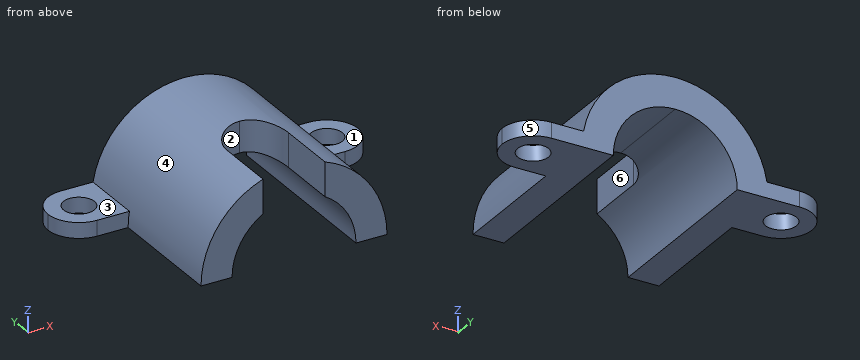
```python
from build123d import *

# Parameters (mm, degrees)
F1_W      = 60
F1_H      = 60
F2_DEPTH  = 30
F4_DEPTH  = 60.001
F5_W      = 20
F5_H      = 20
F6_DEPTH  = 5
F7_W      = 20
F7_H      = 20
F8_DEPTH  = 5
F10_DEPTH = 20
F12_DEPTH = 40
F13_R     = 9.99999
F14_R     = 9.99999
F15_R     = 5
F16_DEPTH = 5.001
F17_R     = 5
F18_DEPTH = 5.001
F20_DEPTH = 30
F21_R     = 10
F22_R     = 9.99999


# Not quite as in the source:
# - a fillet or chamfer is up to 0.001 mm smaller than in the source, because OpenCascade refuses the exact size


with BuildPart() as f2:
    # F1 (on Top) → F2 (new body)
    with BuildSketch(Plane.XY):
        Rectangle(F1_W, F1_H)
    extrude(amount=F2_DEPTH)

    # F3 (on face) → F4 (cut, through all)
    with BuildSketch(Plane.XZ.offset(30)):
        with BuildLine():
            ThreePointArc((20, 0), (14.1421356237, 14.1421356237), (0, 20))
            Line((0, 20), (0, 0))
            Line((0, 0), (20, 0))
        make_face()
        with BuildLine():
            Line((0, 0), (0, 20))
            ThreePointArc((0, 20), (-14.1421356237, 14.1421356237), (-20, 0))
            Line((-20, 0), (0, 0))
        make_face()
    extrude(amount=-F4_DEPTH, mode=Mode.SUBTRACT)

    # F5 (on Top) → F6 (join)
    with BuildSketch(Plane.XY):
        with Locations((40, 20)):
            Rectangle(F5_W, F5_H)
    extrude(amount=F6_DEPTH)

    # F7 (on Top) → F8 (join)
    with BuildSketch(Plane.XY):
        with Locations((-40, 20)):
            Rectangle(F7_W, F7_H)
    extrude(amount=F8_DEPTH)

    # F9 (on face) → F10 (cut)
    with BuildSketch(Plane(origin=(0, 30, 0), x_dir=(-1, 0, 0), z_dir=(0, 1, 0))):
        with BuildLine():
            ThreePointArc((-29.5803989155, 5), (-19.3649167147, 22.9128784886), (4.28e-08, 30))
            Line((4.28e-08, 30), (-30, 30))
            Line((-30, 30), (-30, 5))
            Line((-30, 5), (-29.5803989155, 5))
        make_face()
        with BuildLine():
            ThreePointArc((4.28e-08, 30), (19.3649167474, 22.912878461), (29.5803989155, 5))
            Line((29.5803989155, 5), (30, 5))
            Line((30, 5), (30, 30))
            Line((30, 30), (4.28e-08, 30))
        make_face()
    extrude(amount=-F10_DEPTH, mode=Mode.SUBTRACT)

    # F11 (on face) → F12 (cut)
    with BuildSketch(Plane.XZ.offset(30)):
        with BuildLine():
            Line((-30, 30), (-30, 0))
            ThreePointArc((-30, 0), (-21.2132034683, 21.2132034029), (-9.24e-08, 30))
            Line((-9.24e-08, 30), (-30, 30))
        make_face()
        with BuildLine():
            ThreePointArc((-9.24e-08, 30), (21.2132034029, 21.2132034683), (30, 0))
            Line((30, 0), (30, 30))
            Line((30, 30), (-9.24e-08, 30))
        make_face()
    extrude(amount=-F12_DEPTH, mode=Mode.SUBTRACT)

    # F13 (radius 10 in the source; OpenCascade refuses exactly that, so slightly less here)
    f13_edges = [f2.edges().sort_by_distance(p)[0] for p in [
        (50, 30, 2.5),
        (50, 10, 2.5),
    ]]
    fillet(f13_edges, radius=F13_R)

    # F14 (radius 10 in the source; OpenCascade refuses exactly that, so slightly less here)
    f14_edges = [f2.edges().sort_by_distance(p)[0] for p in [
        (-50, 30, 2.5),
        (-50, 10, 2.5),
    ]]
    fillet(f14_edges, radius=F14_R)

    # F15 (on face) → F16 (cut, through all)
    with BuildSketch(Plane.XY.offset(5)):
        with Locations((-40, 20)):
            Circle(F15_R)
    extrude(amount=-F16_DEPTH, mode=Mode.SUBTRACT)

    # F17 (on face) → F18 (cut, through all)
    with BuildSketch(Plane.XY.offset(5)):
        with Locations((40, 20)):
            Circle(F17_R)
    extrude(amount=-F18_DEPTH, mode=Mode.SUBTRACT)

    # F19 (on face) → F20 (cut)
    with BuildSketch(Plane.XZ.offset(30)):
        with BuildLine():
            Line((10, 17.3205080757), (10, 28.2842712437))
            ThreePointArc((10.0000000012, 28.284271247), (1.3e-09, 30), (-9.9999999988, 28.2842712479))
            Line((-10, 28.2842712513), (-10, 17.3205080757))
            ThreePointArc((-10, 17.3205080757), (0, 20), (10, 17.3205080757))
        make_face()
    extrude(amount=-F20_DEPTH, mode=Mode.SUBTRACT)

    # F21
    f21_edges = [f2.edges().sort_by_distance(p)[0] for p in [
        (-10, 0, 22.80239),
    ]]
    fillet(f21_edges, radius=F21_R)

    # F22 (radius 10 in the source; OpenCascade refuses exactly that, so slightly less here)
    f22_edges = [f2.edges().sort_by_distance(p)[0] for p in [
        (10, 0, 22.80239),
    ]]
    fillet(f22_edges, radius=F22_R)


solid = f2.part
```
Part model, mm, in its own coordinate system. Face numbers are marked on the shaded views. A direction names the side the tool comes from. Round coordinates to 2 decimals unless told otherwise and drop trailing zeros. Loops run counter-clockwise (first coordinate to the right, second up) from the corner with the lowest first, then second, coordinate; pieces in that order, holes last.
1. Slice it at D-D (y = 6.5). Give the cut face in (x, z).
Solutions:
outline: (-30, 0) - (-20, 0) arc R20 cw to (20, 0) - (30, 0) arc R30 ccw to start
2. Slice it at B-B (y = 17). Give the cut face in (x, z), and give its area (3 significant figures).
Solutions:
outline: (-49.54, 0) - (-44, 0) - (-44, 5) - (-49.54, 5) - close; (-36, 0) - (-20, 0) arc R20 cw to (20, 0) - (36, 0) - (36, 5) - (29.58, 5) arc R30 ccw to (-29.58, 5) - (-36, 5) - close; (44, 0) - (49.54, 0) - (49.54, 5) - (44, 5) - close
area: 902 mm2
3. Flat gauge pins, fed straight in: pin 1 (1 mm diameter, centred on y = 4.5, z = 15, fed in from -X); pin 2 (16 mm diameter, centred on x = 40, y = 20, fed in from +Z); pin 3 (10 mm diameter, centred on x = 7, y = 12.5, fed in from +Z); pin 4 (8 mm diameter, centred on x = -40, y = 20, fed in from -Z). Where does each tip first touch, or does it go through?
Solutions:
pin 1: stops at x = -26.26
pin 2: stops at z = 5
pin 3: stops at z = 29.93
pin 4: passes through
4. Slice it at C-C (z = 3). Count the separate pieces of the cut face and the enclosed holes in it, and give its area (3 significant figures).
Solutions:
separate pieces: 2
enclosed holes: 2
area: 1,770 mm2
5. Slice it at A-A (z = 9). Give the cut face in (x, y).
Solutions:
outline: (-28.62, -30) - (-17.86, -30) - (-17.86, 30) - (-28.62, 30) - close; (17.86, -30) - (28.62, -30) - (28.62, 30) - (17.86, 30) - close
6. Drill centre lines: line 1 along Y through (x, z) = (40, 3); line 2 along X through (y, z) = (14, 3); line 3 along X through (y, z) = (18.5, 9). Where is each one in solid material? Low to high.
Solutions:
line 1: y = 10 to 15, 25 to 30
line 2: x = -48 to -19.77, 19.77 to 48
line 3: x = -28.62 to -17.86, 17.86 to 28.62
7. 3-axis set-ups, long thin cutter, end or side, ignore diameter. For the marked faces 1, 2 and 3: which of +Z, -Z, +X, -X, +Y, -Y reach the whole face in a straight line?
Solutions:
face 1: +Z, +X, +Y, -Y
face 2: +Z, -Z, -Y
face 3: +Z, -X, +Y, -Y
8. Two-plate mould, pull along X, no slides. Class the marked faces 4, 5 and 6: pulls with the +X half, pulls with the -X half, needs draft (parallel to the pull), parting line crosses it, or undercut.
Solutions:
face 4: parting line crosses it
face 5: pulls with the +X half
face 6: undercut
